```python
from build123d import *

# Parameters (mm, degrees)
F0_W     = 31.75
F0_H     = 63.5
F0_R     = 6.35
F1_DEPTH = 6.35


with BuildPart() as f1:
    # F0 (on Top) → F1 (new body)
    with BuildSketch(Plane.XY):
        Rectangle(F0_W, F0_H)
        with BuildLine():
            ThreePointArc((3.175, -15.46225), (6.289466, -20.8915), (3.175, -26.32075))
            Line((3.175, -26.32075), (-3.175, -26.32075))
            ThreePointArc((-3.175, -26.32075), (-6.289466, -20.8915), (-3.175, -15.46225))
            Line((-3.175, -15.46225), (3.175, -15.46225))
        make_face(mode=Mode.SUBTRACT)
        with Locations((0, 20.6375)):
            Circle(F0_R, mode=Mode.SUBTRACT)
    extrude(amount=F1_DEPTH)


solid = f1.part
```
CAD build for the part. Positions are in the model's coordinates, mm. A direction names the side the tool comes from. Round coordinates to 2 decimals unless told otherwise and drop trailing zeros. Order: outer loops, then holes, each group sorted by start corner. A loop starts at its lowest first (then second) coordinate and runs counter-clockwise, first axis right, second up.
Item 1: Saw through at C-C on z = 2.25. State how many separate pieces and enclosed holes the cut face has, then the cut area to 3 significant figures.
Item 2: Saw through at B-B on y = 16. Write the cut outline in (x, z) (3 decimals), then the cut area to 3 significant figures.
Item 3: Tool access for faces 1 (the face through (0, -26.321, 3)), 2 (the face through (0, 31.75, 3)): list every direction of +Z, -Z, +X, -X, +Y, -Y with a clear straight run to the whole face (end or side of a thin tool).
Item 4: Saw through at A-A on x = 0. Write the cut outline in (y, z), then the cut area to 3 significant figures.
Item 5: Mould opens along Y. For faces 3 (the face through (0, 0, 6.35)), 4 (the face through (6.29, -20.8, 3.13)), 5 (the face through (0, -31.75, 3)) say: pulls with the +Y half, pulls with the -Y half, needs draft (parallel to the pull), parting line crosses it, or undercut.
Item 6: Probe line 1 along Y through (x, z) = (0, 5.25); line 2 along Y through (x, z) = (5, 2.25); line 3 along X through (y, z) = (-22, 3.25) (3 decimals). List the from-to ranges inside material, lowest first.
Reported:
1. separate pieces: 1
1. enclosed holes: 2
1. area: 1,770 mm2
2. outline: (-15.875, 0) - (-4.338, 0) - (-4.338, 6.35) - (-15.875, 6.35) - close; (4.338, 0) - (15.875, 0) - (15.875, 6.35) - (4.338, 6.35) - close
2. area: 147 mm2
3. face 1: +Z, -Z
3. face 2: +Z, -Z, +X, -X, +Y
4. outline: (-31.75, 0) - (-26.32, 0) - (-26.32, 6.35) - (-31.75, 6.35) - close; (-15.46, 0) - (14.29, 0) - (14.29, 6.35) - (-15.46, 6.35) - close; (26.99, 0) - (31.75, 0) - (31.75, 6.35) - (26.99, 6.35) - close
4. area: 254 mm2
5. face 3: needs draft
5. face 4: undercut
5. face 5: pulls with the -Y half
6. line 1: y = -31.75 to -26.32, -15.46 to 14.29, 26.99 to 31.75
6. line 2: y = -31.75 to -24.71, -17.08 to 16.72, 24.55 to 31.75
6. line 3: x = -15.875 to -6.191, 6.191 to 15.875
